from build123d import *

# Parameters (mm, degrees)
EXTRUDE_1_DEPTH             = 2.8
EXTRUDE_2_DEPTH             = 4.5
SKETCH_2_R                  = 1.5
CUT_EXTRUDE_1_DEPTH         = 5
PATTERN_LINEAR_1_COUNT      = 2
PATTERN_LINEAR_1_PITCH      = 142
PATTERN_LINEAR_1_COUNT_DIR2 = 2
PATTERN_LINEAR_1_PITCH_DIR2 = 54
CUT_EXTRUDE_2_DEPTH         = 2
SKETCH_7_R                  = 1.5
CUT_EXTRUDE_3_DEPTH         = 3
SKETCH_8_W                  = 7
SKETCH_8_H                  = 7
CUT_EXTRUDE_4_DEPTH         = 5
EXTRUDE_3_DEPTH             = 56
FILLET_1_R                  = 2


with BuildPart() as part:
    # Sketch 1 → Extrude 1 (new body)
    with BuildSketch(Plane.XY):
        with BuildLine():
            Line((-71, -34.5), (71, -34.5))
            ThreePointArc((71, -34.5), (76.303300859, -32.303300859), (78.5, -27))
            Line((78.5, -27), (78.5, 27))
            ThreePointArc((78.5, 27), (76.303300859, 32.303300859), (71, 34.5))
            Line((71, 34.5), (-71, 34.5))
            ThreePointArc((-71, 34.5), (-76.303300859, 32.303300859), (-78.5, 27))
            Line((-78.5, 27), (-78.5, -27))
            ThreePointArc((-78.5, -27), (-76.303300859, -32.303300859), (-71, -34.5))
        make_face()
        with BuildLine():
            Line((-71, -33), (71, -33))
            ThreePointArc((71, -33), (75.242640687, -31.242640687), (77, -27))
            Line((77, -27), (77, 27))
            ThreePointArc((77, 27), (75.242640687, 31.242640687), (71, 33))
            Line((71, 33), (-71, 33))
            ThreePointArc((-71, 33), (-75.242640687, 31.242640687), (-77, 27))
            Line((-77, 27), (-77, -27))
            ThreePointArc((-77, -27), (-75.242640687, -31.242640687), (-71, -33))
        make_face(mode=Mode.SUBTRACT)
    extrude(amount=-EXTRUDE_1_DEPTH)

    # Sketch 1_2 → Extrude 2 (add)
    with BuildSketch(Plane.XY):
        with BuildLine():
            Line((-71, 33), (71, 33))
            ThreePointArc((71, 33), (75.242640687, 31.242640687), (77, 27))
            Line((77, 27), (77, -27))
            ThreePointArc((77, -27), (75.242640687, -31.242640687), (71, -33))
            Line((71, -33), (-71, -33))
            ThreePointArc((-71, -33), (-75.242640687, -31.242640687), (-77, -27))
            Line((-77, -27), (-77, 27))
            ThreePointArc((-77, 27), (-75.242640687, 31.242640687), (-71, 33))
        make_face()
    extrude(amount=-EXTRUDE_2_DEPTH)

    # Sketch 2 → Cut-Extrude 1 (cut)
    with BuildSketch(Plane.XY):
        with Locations((-71, 27)):
            Circle(SKETCH_2_R)
        with Locations((-71, -27)):
            Circle(SKETCH_2_R)
        with Locations((71, 27)):
            Circle(SKETCH_2_R)
        with Locations((71, -27)):
            Circle(SKETCH_2_R)
        with Locations((-17, -27)):
            Circle(SKETCH_2_R)
    extrude(amount=-CUT_EXTRUDE_1_DEPTH, mode=Mode.SUBTRACT)

    # Sketch 4 → Cut-Revolve 1 (revolve, cut)
    with BuildSketch(Plane(origin=(-71, 0, 0), x_dir=(0, 0, -1), z_dir=(1, 0, 0)), mode=Mode.PRIVATE) as cut_revolve_1_sk:
        Polygon((2.75, 27), (0, 27), (0, 29.75), align=None)
    cut_revolve_1 = revolve(cut_revolve_1_sk.sketch.rotate(Axis((-71, 27, 0.2), (0, 0, -1)), 90), axis=Axis((-71, 27, 0.2), (0, 0, -1)), mode=Mode.SUBTRACT)

    # Pattern Linear 1: Cut-Revolve 1 2 × 2
    with Locations(*[(i * PATTERN_LINEAR_1_PITCH, -j * PATTERN_LINEAR_1_PITCH_DIR2, 0) for i in range(PATTERN_LINEAR_1_COUNT) for j in range(PATTERN_LINEAR_1_COUNT_DIR2) if (i, j) != (0, 0)]):
        add(cut_revolve_1, mode=Mode.SUBTRACT)

    # Sketch 5 → Cut-Revolve 2 (revolve, cut)
    with BuildSketch(Plane(origin=(-17, 0, 0), x_dir=(0, 0, -1), z_dir=(1, 0, 0)), mode=Mode.PRIVATE) as cut_revolve_2_sk:
        Polygon((2.75, -27), (0, -27), (0, -24.25), align=None)
    revolve(cut_revolve_2_sk.sketch.rotate(Axis((-17, -27, 0.2), (0, 0, -1)), 90), axis=Axis((-17, -27, 0.2), (0, 0, -1)), mode=Mode.SUBTRACT)

    # Sketch 6 → Cut-Extrude 2 (cut)
    with BuildSketch(Plane.XY):
        with BuildLine():
            Line((-71, -21.75), (-54.5, -21.75))
            ThreePointArc((-54.5, -21.75), (-52.555456352, -22.555456352), (-51.75, -24.5))
            Line((-51.75, -24.5), (-51.75, -27))
            ThreePointArc((-51.75, -27), (-52.555456352, -28.944543648), (-54.5, -29.75))
            Line((-54.5, -29.75), (-71, -29.75))
            ThreePointArc((-71, -29.75), (-72.944543648, -28.944543648), (-73.75, -27))
            Line((-73.75, -27), (-73.75, -24.5))
            ThreePointArc((-73.75, -24.5), (-72.944543648, -22.555456352), (-71, -21.75))
        make_face()
    extrude(amount=-CUT_EXTRUDE_2_DEPTH, mode=Mode.SUBTRACT)

    # Sketch 7 → Cut-Extrude 3 (cut)
    with BuildSketch(Plane.XY.offset(-2)):
        with Locations((-71, -27)):
            Circle(SKETCH_7_R)
        with BuildLine():
            Line((-65.5, -22.8), (-56.5, -22.8))
            ThreePointArc((-56.5, -22.8), (-54.3, -25), (-56.5, -27.2))
            Line((-56.5, -27.2), (-65.5, -27.2))
            ThreePointArc((-65.5, -27.2), (-67.7, -25), (-65.5, -22.8))
        make_face()
    extrude(amount=-CUT_EXTRUDE_3_DEPTH, mode=Mode.SUBTRACT)

    # Sketch 8 → Cut-Extrude 4 (cut)
    with BuildSketch(Plane.XY):
        with Locations((-19, 24)):
            Rectangle(SKETCH_8_W, SKETCH_8_H)
        with Locations((-19, 15)):
            Rectangle(SKETCH_8_W, SKETCH_8_H)
        with Locations((-19, 6.5)):
            Rectangle(SKETCH_8_W, SKETCH_8_H)
    extrude(amount=-CUT_EXTRUDE_4_DEPTH, mode=Mode.SUBTRACT)

    # Sketch 9 → Extrude 3 (add)
    with BuildSketch(Plane(origin=(55, 0, 0), x_dir=(0, 0, -1), z_dir=(1, 0, 0))):
        Polygon((17.5, -24), (4.5, -24), (4.5, -28.5), (19.5, -28.5), (19.5, 28.5), (4.5, 28.5), (4.5, 24), (17.5, 24), align=None)
    extrude(amount=-EXTRUDE_3_DEPTH)

    # Fillet 1
    fillet_1_edges = [part.edges().sort_by_distance(p)[0] for p in [
        (27, 28.5, -19.5),
        (27, -28.5, -19.5),
    ]]
    fillet(fillet_1_edges, radius=FILLET_1_R)


solid = part.part
The model under review builds one solid part; all positions refer to its coordinate system, in mm. A direction names the side the tool comes from. Give positions to 0.01 mm unless a question says otherwise; leave off trailing zeros. Order: outer loops, then holes, each group sorted by start corner. A loop starts at its lowest first (then second) coordinate and runs counter-clockwise, first axis right, second up. Notation, with made-up numbers: M -37.75,28 L -18.75,28 A20 ccw -18.75,51 Z; hole C 31,-27 d2. An arc over 180 degrees is marked long. Answer in a Markdown table with one row per item. Add a question column.
1. Add section B-B on x = -17. State the section outline as (y, z) points, plus the area to 3 significant figures.
2. Machinability: for faces 1 (the flat face through (-1, -2, -18)), 2 (the cylindrical face through (-52.58, -22.53, -0.99)), 3 (the flat face through (27, -24, -11)), 4 (the flat face through (-19, 10, -2)), which of the approach directions +Z, -Z, +X, -X, +Y, -Y give a long, thin tool a straight path to every point of the face, cutting with its end or side? Answer none if there is none.
3. Add section C-C on y = 22.5. State the section outline as (x, z) points.
4. For pin 1 Ø4 at (x, y) = (71, 27) entering from +Z; pin 2 Ø10.5 at (x, z) = (17, -9.5) entering from +Y; pin 3 Ø6.5 at (x, z) = (25, -13.5) entering from -Y, all flat-tipped, find the tip position at first contact; note any pin that passes through.
5. To check wall thickness, follow line 1 along Y through (x, z) = (71, -2.2); line 2 along X through (y, z) = (27, -2.7); line 3 along X through (y, z) = (27, -3.8). State the ranges of each line that lie inside material, in increasing order.
6. Add section D-D on x = 1.5. State the section outline as (y, z) points.
7. Mouldability with a two-part tool opening along X and no side actions: class faces 5 (the flat face through (27, 28.5, -11)), 6 (the flat face through (-19, 18.5, -2)), 7 (the cylindrical face through (-75.289, 31.196, -3.638)) as released by +X, released by -X, zero draft, split by the parting line, or undercut.
8. Add section A-A on z = -6.5. State the section outline as (x, y) points.
The answers:
| question | item | result |
|---|---|---|
| 1 | outline | M -34.5,-2.8 L -33,-2.8 L -33,-4.5 L -28.5,-4.5 L -28.5,-1.25 L -29.75,0 L -34.5,0 Z; M -25.5,-4.5 L 3,-4.5 L 3,0 L -24.25,0 L -25.5,-1.25 Z; M 10,-4.5 L 11.5,-4.5 L 11.5,0 L 10,0 Z; M 18.5,-4.5 L 20.5,-4.5 L 20.5,0 L 18.5,0 Z; M 27.5,-4.5 L 33,-4.5 L 33,-2.8 L 34.5,-2.8 L 34.5,0 L 27.5,0 Z |
| 1 | area | 196 mm2 |
| 2 | face 1 | -Z, -X, +Y, -Y |
| 2 | face 2 | +Z |
| 2 | face 3 | +X, -X |
| 2 | face 4 | +Z, -Z |
| 3 | outline | M -78.5,-2.8 L -77,-2.8 L -77,-4.5 L -22.5,-4.5 L -22.5,0 L -78.5,0 Z; M -15.5,-4.5 L 77,-4.5 L 77,-2.8 L 78.5,-2.8 L 78.5,0 L -15.5,0 Z; M -1,-19.5 L 55,-19.5 L 55,-17.5 L -1,-17.5 Z |
| 4 | pin 1 | z = -0.75 |
| 4 | pin 2 | y = 33 |
| 4 | pin 3 | y = -28.5 |
| 5 | line 1 | -34.5 to -28.5, -25.5 to 25.5, 28.5 to 34.5 |
| 5 | line 2 | -78.5 to -72.5, -69.5 to -22.5, -15.5 to 69.5, 72.5 to 78.5 |
| 5 | line 3 | -77 to -72.5, -69.5 to -22.5, -15.5 to 69.5, 72.5 to 77 |
| 6 | outline | M -34.5,-2.8 L -33,-2.8 L -33,-4.5 L -28.5,-4.5 L -28.5,-17.5 A2 ccw -26.5,-19.5 L 26.5,-19.5 A2 ccw 28.5,-17.5 L 28.5,-4.5 L 33,-4.5 L 33,-2.8 L 34.5,-2.8 L 34.5,0 L -34.5,0 Z; hole M -24,-17.5 L 24,-17.5 L 24,-4.5 L -24,-4.5 Z |
| 7 | face 5 | zero draft |
| 7 | face 6 | undercut |
| 7 | face 7 | released by -X |
| 8 | outline | M -1,-28.5 L 55,-28.5 L 55,-24 L -1,-24 Z; M -1,24 L 55,24 L 55,28.5 L -1,28.5 Z |
